Read the model definition and answer for the solid it produces. Units are mm, in the model's axes. Face numbers are marked on the shaded views. Give positions to 0.01 mm unless a question says otherwise; leave off trailing zeros. Write each loop counter-clockwise with the first axis right and the second up, starting at its lowest first coordinate (ties: lowest second). Pieces come first, ordered by that corner, then holes. Notation, with made-up numbers: (43.25, 75) -> (54.25, 75) arc R34 ccw to (54.25, 106) -> close; hole circle Ø10 at (77, 65). An arc over 180 degrees is marked (long way). Answer as CSV lines item,"result". Start each with the question number.
1. The part is cut by section C-C, the plane y = 0.5. Determine the outline of the cut face in (x, z).
2. For a pull along Z with two mould halves and no side action, classify the marked faces 1, 2, 3 and 4 as pulls with the +Z half, pulls with the -Z half, needs draft (parallel to the pull), parting line crosses it, or undercut.
3. Find the intervals of material crossed by line 1 (X direction, y = -2, z = -31.75); line 2 (Z direction, x = -2, y = 2.5); line 3 (X direction, y = -1.5, z = 34), in increasing order.
4. The part is cut by section A-A, the plane z = 31.75. Determine the outline of the cut face in (x, y), and give its area (3 significant figures).
5. The part is cut by section B-B, the plane x = 0. Determine the outline of the cut face in (y, z), and give its area (3 significant figures).
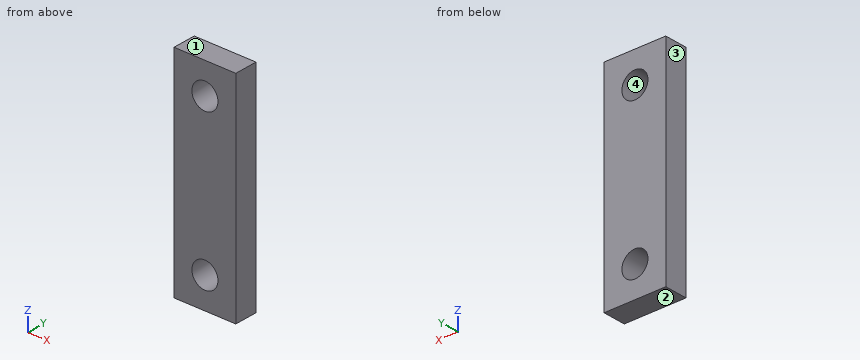
from build123d import *

# Parameters (mm, degrees)
SKETCH1_W                   = 25.4
SKETCH1_H                   = 9.525
EXTRUDE1_DEPTH              = 44.45
TAP_DRILL_FOR_1_2_13_TAP1_D = 10.71626


with BuildPart() as part:
    # Sketch1 → Extrude1 (new body, symmetric)
    with BuildSketch(Plane.XY):
        Rectangle(SKETCH1_W, SKETCH1_H)
    extrude(amount=EXTRUDE1_DEPTH, both=True)

    # Tap Drill for 1/2-13 Tap1 (through all)
    with Locations(Plane(origin=(0, 4.7625, -31.75), x_dir=(0, 0, 1), z_dir=(0, 1, 0))):
        with Locations((0, 0)):
            tap_drill_for_1_2_13_tap1 = Hole(TAP_DRILL_FOR_1_2_13_TAP1_D / 2)

    # Mirror1: Tap Drill for 1/2-13 Tap1 across plane
    add(tap_drill_for_1_2_13_tap1.mirror(Plane.XY), mode=Mode.SUBTRACT)


solid = part.part
Results found:
1,outline,"(-12.7, -44.45) -> (12.7, -44.45) -> (12.7, 44.45) -> (-12.7, 44.45) -> close; hole circle Ø10.72 at (0, -31.75); hole circle Ø10.72 at (0, 31.75)"
2,face 1,"pulls with the +Z half"
2,face 2,"pulls with the -Z half"
2,face 3,"needs draft"
2,face 4,"undercut"
3,line 1,"x = -12.7 to -5.36, 5.36 to 12.7"
3,line 2,"z = -44.45 to -36.72, -26.78 to 26.78, 36.72 to 44.45"
3,line 3,"x = -12.7 to -4.86, 4.86 to 12.7"
4,outline,"(-12.7, -4.76) -> (-5.36, -4.76) -> (-5.36, 4.76) -> (-12.7, 4.76) -> close; (5.36, -4.76) -> (12.7, -4.76) -> (12.7, 4.76) -> (5.36, 4.76) -> close"
4,area,"140 mm²"
5,outline,"(-4.76, -44.45) -> (4.76, -44.45) -> (4.76, -37.11) -> (-4.76, -37.11) -> close; (-4.76, -26.39) -> (4.76, -26.39) -> (4.76, 26.39) -> (-4.76, 26.39) -> close; (-4.76, 37.11) -> (4.76, 37.11) -> (4.76, 44.45) -> (-4.76, 44.45) -> close"
5,area,"643 mm²"
